Part model, mm, in its own coordinate system. Face numbers are marked on the shaded views. A direction names the side the tool comes from. Give positions to 0.01 mm unless a question says otherwise; leave off trailing zeros. Write each loop counter-clockwise with the first axis right and the second up, starting at its lowest first coordinate (ties: lowest second). Pieces come first, ordered by that corner, then holes. Notation, with made-up numbers: M 27.25,-39.75 L 54.25,-39.75 A19 cw 54.25,-15.75 Z; hole C 34,13 d7. An arc over 180 degrees is marked long. Use a Markdown table: item, result. Add a question column.
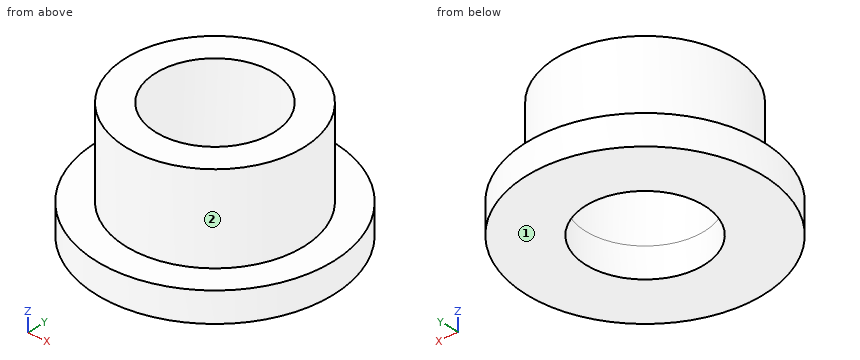
from build123d import *

# Parameters (mm, degrees)
F0_R     = 6.31
F1_DEPTH = 1.59
F2_R     = 3.15
F3_DEPTH = 1.591
F4_R     = 4.74
F4_R_2   = 3.15
F5_DEPTH = 4.71


with BuildPart() as f1:
    # F0 (on Top) → F1 (new body)
    with BuildSketch(Plane.XY):
        Circle(F0_R)
    extrude(amount=F1_DEPTH)

    # F2 (on face) → F3 (cut, through all)
    with BuildSketch(Plane.XY.offset(1.59)):
        Circle(F2_R)
    extrude(amount=-F3_DEPTH, mode=Mode.SUBTRACT)

    # F4 (on face) → F5 (join)
    with BuildSketch(Plane.XY.offset(1.59)):
        Circle(F4_R)
        Circle(F4_R_2, mode=Mode.SUBTRACT)
    extrude(amount=F5_DEPTH)


solid = f1.part
1. Cut at C-C (y = 3.5). Write the cut outline in (x, z), then the cut area to 3 significant figures.
2. Cut at D-D (x = 5). Write the cut outline in (y, z).
3. Flat gauge pins, fed straight in: pin 1 (3 mm diameter, centred on y = 2, z = 2.5, fed in from -X); pin 2 (1.5 mm diameter, centred on y = -4, z = 3.5, fed in from -X). Where does each tip first touch, or does it go through?
4. Tool access for the marked faces 1 and 2: list every direction of +Z, -Z, +X, -X, +Y, -Y with a clear straight run to the whole face (end or side of a thin tool).
5. Cut at A-A (y = 0). Write the cut outline in (x, z).
6. Drill centre lines: probe 1 along Y at (x, z) = (0, 2.7); probe 2 along Y at (x, z) = (0, 0.35); probe 3 along Z at (x, y) = (2.25, 5.5). Where is each one in solid material? Low to high. Write a range as [from, to].
A:
| question | item | result |
|---|---|---|
| 1 | outline | M -5.25,0 L 5.25,0 L 5.25,1.59 L 3.2,1.59 L 3.2,6.3 L -3.2,6.3 L -3.2,1.59 L -5.25,1.59 Z |
| 1 | area | 46.8 mm² |
| 2 | outline | M -3.85,0 L 3.85,0 L 3.85,1.59 L -3.85,1.59 Z |
| 3 | pin 1 | stops at x = -6.26 |
| 3 | pin 2 | stops at x = -3.45 |
| 4 | face 1 | -Z, +X, -X, +Y, -Y |
| 4 | face 2 | +Z |
| 5 | outline | M -6.31,0 L -3.15,0 L -3.15,6.3 L -4.74,6.3 L -4.74,1.59 L -6.31,1.59 Z; M 3.15,0 L 6.31,0 L 6.31,1.59 L 4.74,1.59 L 4.74,6.3 L 3.15,6.3 Z |
| 6 | probe 1 | y = [-4.74, -3.15], [3.15, 4.74] |
| 6 | probe 2 | y = [-6.31, -3.15], [3.15, 6.31] |
| 6 | probe 3 | z = [0, 1.59] |
